Part model, mm, in its own coordinate system. A direction names the side the tool comes from. Coordinates: 2 decimals unless noted, no trailing zeros. Order: outer loops, then holes, each group sorted by start corner. A loop starts at its lowest first (then second) coordinate and runs counter-clockwise, first axis right, second up.
from build123d import *

# Parameters (mm, degrees)
BOSS_EXTRUDE1_DEPTH     = 15
CUT_EXTRUDE1_DEPTH      = 30
SKETCH3_R               = 1.5
CUT_EXTRUDE2_DEPTH      = 30
MIRROR2_COPY_1_DEPTH    = 30
MIRROR2_COPY_2_SKETCH_R = 1.5
MIRROR2_COPY_2_DEPTH    = 30
SKETCH4_R               = 1.5
CUT_EXTRUDE3_DEPTH      = 5


with BuildPart() as part:
    # Sketch1 → Boss-Extrude1 (new body)
    with BuildSketch(Plane.XY):
        with BuildLine():
            Line((12, 0), (-12, 0))
            ThreePointArc((-12, 0), (-15, 3), (-18, 0))
            Line((-18, 0), (-24, 0))
            ThreePointArc((-24, 0), (-16.521917809, 8.870387037), (-6.514718626, 3))
            Line((-6.514718626, 3), (6.514718626, 3))
            ThreePointArc((6.514718626, 3), (16.521917809, 8.870387037), (24, 0))
            Line((24, 0), (18, 0))
            ThreePointArc((18, 0), (15, 3), (12, 0))
        make_face()
    extrude(amount=BOSS_EXTRUDE1_DEPTH)

    # Sketch2 → Cut-Extrude1 (cut)
    with BuildSketch(Plane(origin=(0, 2, 0), x_dir=(-1, 0, 0), z_dir=(0, -1, 0))):
        Polygon((-20.5, -10.675426481), (-17.75, -9.08771324), (-17.75, -5.91228676), (-20.5, -4.324573519), (-23.25, -5.91228676), (-23.25, -9.08771324), align=None)
    cut_extrude1 = extrude(amount=-CUT_EXTRUDE1_DEPTH, mode=Mode.SUBTRACT)

    # Sketch3 → Cut-Extrude2 (cut)
    with BuildSketch(Plane(origin=(0, 2, 0), x_dir=(1, 0, 0), z_dir=(0, 1, 0))):
        with Locations(Location((20.5, -7.5, 0), (0, 0, 180))):
            Circle(SKETCH3_R)
    cut_extrude2 = extrude(amount=-CUT_EXTRUDE2_DEPTH, mode=Mode.SUBTRACT)

    # Mirror1: Cut-Extrude1, Cut-Extrude2 across plane
    add(cut_extrude1.mirror(Plane.ZY.offset(-15)), mode=Mode.SUBTRACT)
    add(cut_extrude2.mirror(Plane.ZY.offset(-15)), mode=Mode.SUBTRACT)

    # Mirror2: Cut-Extrude1, Cut-Extrude2 across plane
    add(cut_extrude1.mirror(Plane(origin=(0, 0, 0), x_dir=(0, 0, 1), z_dir=(1, 0, 0))), mode=Mode.SUBTRACT)
    add(cut_extrude2.mirror(Plane(origin=(0, 0, 0), x_dir=(0, 0, 1), z_dir=(1, 0, 0))), mode=Mode.SUBTRACT)

    # Mirror2 copy 1 sketch → Mirror2 copy 1 (cut)
    with BuildSketch(Plane(origin=(-30, 2, 0), x_dir=(-1, 0, 0), z_dir=(0, -1, 0))):
        Polygon((-20.5, -10.675426481), (-17.75, -9.08771324), (-17.75, -5.91228676), (-20.5, -4.324573519), (-23.25, -5.91228676), (-23.25, -9.08771324), align=None)
    extrude(amount=-MIRROR2_COPY_1_DEPTH, mode=Mode.SUBTRACT)

    # Mirror2 copy 2 sketch → Mirror2 copy 2 (cut)
    with BuildSketch(Plane(origin=(-30, 2, 0), x_dir=(1, 0, 0), z_dir=(0, 1, 0))):
        with Locations(Location((20.5, -7.5, 0), (0, 0, 180))):
            Circle(MIRROR2_COPY_2_SKETCH_R)
    extrude(amount=-MIRROR2_COPY_2_DEPTH, mode=Mode.SUBTRACT)

    # Sketch4 → Cut-Extrude3 (cut)
    with BuildSketch(Plane(origin=(0, 3, 0), x_dir=(1, 0, 0), z_dir=(0, 1, 0))):
        with Locations(Location((0, -7.5, 0), (0, 0, 270))):
            Circle(SKETCH4_R)
    extrude(amount=-CUT_EXTRUDE3_DEPTH, mode=Mode.SUBTRACT)


solid = part.part
Q1. Cut at B-B on z = 11.25. Write the cut outline in (x, y), and give its area (3 significant figures).
Results list:
outline: (-24, 0) - (-18, 0) arc R3 cw to (-12, 0) - (12, 0) arc R3 cw to (18, 0) - (24, 0) arc R9 ccw to (6.51, 3) - (-6.51, 3) arc R9 ccw to start
area: 263 mm2
Q2. Cut at C-C on x = 1. Write the cut outline in (y, z).
Results list:
outline: (0, 0) - (3, 0) - (3, 6.38) - (0, 6.38) - close; (0, 8.62) - (3, 8.62) - (3, 15) - (0, 15) - close
Q3. Cut at A-A on y = 1.25. Write the cut outline in (x, z).
Results list:
outline: (-23.91, 0) - (-17.73, 0) - (-17.73, 15) - (-23.91, 15) - close; (-12.27, 0) - (12.27, 0) - (12.27, 15) - (-12.27, 15) - close; (17.73, 0) - (23.91, 0) - (23.91, 15) - (17.73, 15) - close; hole circle Ø3 at (-20.5, 7.5); hole circle Ø3 at (-9.5, 7.5); hole circle Ø3 at (0, 7.5); hole circle Ø3 at (9.5, 7.5); hole circle Ø3 at (20.5, 7.5)
Q4. Wall check: line 1 along X through (y, z) = (4.5, 8); line 2 along Z through (x, y) = (20.5, 0.45); line 3 along X through (y, z) = (6.25, 4.5). Give the ranges that are in metal, low to high.
Results list:
line 1: x = -17.75 to -12.25, 12.25 to 17.75
line 2: z = 0 to 6, 9 to 15
line 3: x = -21.48 to -20.8, -20.2 to -9.8, -9.2 to -8.52, 8.52 to 9.2, 9.8 to 20.2, 20.8 to 21.48
Q5. Pin check, flat tips, straight feed: pin 1 Ø1.8 at (x, z) = (20.5, 7.5) entering from -Y; pin 2 Ø1 at (y, z) = (5.5, 7) entering from -X; pin 3 Ø1.6 at (x, z) = (-19.5, 8.5) entering from +Y; pin 4 Ø1.6 at (y, z) = (4, 8) entering from -X. Stop position of each tip, or through.
Results list:
pin 1: passes through
pin 2: stops at x = -17.75
pin 3: stops at y = 2
pin 4: stops at x = -23.41
Q6. Mould opens along Z. For faces 1 (the face through (17.75, 5, 8)), 2 (the face through (-15, 3, 7)), 3 (the face through (0.3, 2.6, 15)) say: pulls with the +Z half, pulls with the -Z half, needs draft (parallel to the pull), parting line crosses it, or undercut.
Results list:
face 1: undercut
face 2: needs draft
face 3: pulls with the +Z half
Q7. Which spindle directions (+Z, -Z, +X, -X, +Y, -Y) get a long thin tool onto all of the face, cutting with end or side? Do faces 4 (the face through (23.25, 3, 7)), 5 (the face through (-16.7, 8.84, 7.4)). Say none if no direction does.
Results list:
face 4: +Y
face 5: +Z, -Z, +Y
